The model under review builds one solid part; all positions refer to its coordinate system, in mm. Face numbers are marked on the shaded views. A direction names the side the tool comes from. Give positions to 0.01 mm unless a question says otherwise; leave off trailing zeros. Write each loop counter-clockwise with the first axis right and the second up, starting at its lowest first coordinate (ties: lowest second). Pieces come first, ordered by that corner, then holes. Notation, with made-up numbers: (-26.75, 31.25) - (7.25, 31.25) arc R24 ccw to (7.25, 67.25) - close; hole circle Ø3 at (8, 46.5). An arc over 180 degrees is marked (long way). Write item = value, one per line.
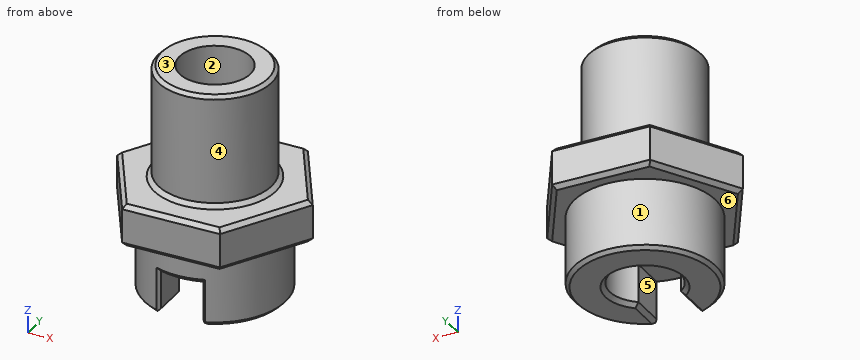
```python
from build123d import *

# Parameters (mm, degrees)
SKETCH1_R           = 4
BOSS_EXTRUDE1_DEPTH = 8
BOSS_EXTRUDE2_DEPTH = 3
SKETCH3_R           = 5
BOSS_EXTRUDE3_DEPTH = 5
SKETCH4_R           = 2.5
CUT_EXTRUDE1_DEPTH  = 19.439088915
CHAMFER1_SIZE       = 0.3
CHAMFER2_SIZE       = 0.3
SKETCH5_W           = 3
SKETCH5_H           = 3
CUT_EXTRUDE2_DEPTH  = 13.165525061
CHAMFER3_SIZE       = 0.3
CHAMFER4_SIZE       = 0.3
CHAMFER5_SIZE       = 0.25


with BuildPart() as part:
    # Sketch1 → Boss-Extrude1 (new body)
    with BuildSketch(Plane.XY):
        Circle(SKETCH1_R)
    extrude(amount=BOSS_EXTRUDE1_DEPTH)

    # Sketch2 → Boss-Extrude2 (add)
    with BuildSketch(Plane(origin=(0, 0, 0), x_dir=(-1, 0, 0), z_dir=(0, 0, -1))):
        Polygon((-3.464101615, 6), (-6.92820323, 0), (-3.464101615, -6), (3.464101615, -6), (6.92820323, 0), (3.464101615, 6), align=None)
    extrude(amount=BOSS_EXTRUDE2_DEPTH)

    # Sketch3 → Boss-Extrude3 (add)
    with BuildSketch(Plane(origin=(0, 0, -3), x_dir=(-1, 0, 0), z_dir=(0, 0, -1))):
        Circle(SKETCH3_R)
    extrude(amount=BOSS_EXTRUDE3_DEPTH)

    # Sketch4 → Cut-Extrude1 (cut, through all)
    with BuildSketch(Plane.XY.offset(8)):
        Circle(SKETCH4_R)
    extrude(amount=-CUT_EXTRUDE1_DEPTH, mode=Mode.SUBTRACT)

    # Chamfer1
    chamfer1_edges = [part.edges().sort_by_distance(p)[0] for p in [
        (-4, 0, 0),
    ]]
    chamfer(chamfer1_edges, length=CHAMFER1_SIZE)

    # Chamfer2
    chamfer2_edges = [part.edges().sort_by_distance(p)[0] for p in [
        (-2.5, 0, -8),
    ]]
    chamfer(chamfer2_edges, length=CHAMFER2_SIZE)

    # Sketch5 → Cut-Extrude2 (cut, through all)
    with BuildSketch(Plane(origin=(0, 0, 0), x_dir=(1, 0, 0), z_dir=(0, 1, 0))):
        with Locations((0, 6.5)):
            Rectangle(SKETCH5_W, SKETCH5_H)
    extrude(amount=-CUT_EXTRUDE2_DEPTH, mode=Mode.SUBTRACT)

    # Chamfer3
    chamfer3_edges = [part.edges().sort_by_distance(p)[0] for p in [
        (-5.196152423, 3, -3),
        (0, 6, 0),
        (5.196152423, 3, 0),
        (5.196152423, -3, 0),
        (0, -6, 0),
        (-5.196152423, -3, 0),
        (-5.196152423, 3, 0),
        (0, 6, -3),
        (5.196152423, 3, -3),
        (5.196152423, -3, -3),
        (0, -6, -3),
        (-5.196152423, -3, -3),
    ]]
    chamfer(chamfer3_edges, length=CHAMFER3_SIZE)

    # Chamfer4
    # the kernel refuses this chamfer: 0.3, 0.239246049 mm, written as the material it takes off along each edge
    with BuildSketch(Plane(origin=(1.5, -1.592813187, -8), x_dir=(0, 0, 1), z_dir=(0, -1, 0))) as chamfer4_piece_1:
        Polygon((CHAMFER4_SIZE, 0), (0, -CHAMFER4_SIZE), (0, 0), align=None)
    extrude(amount=3.948387716, mode=Mode.SUBTRACT)
    with BuildSketch(Plane(origin=(-1.5, -1.592813187, -8), x_dir=(0, 0, 1), z_dir=(0, -1, 0))) as chamfer4_piece_2:
        Polygon((CHAMFER4_SIZE, 0), (0, CHAMFER4_SIZE), (0, 0), align=None)
    extrude(amount=3.948387716, mode=Mode.SUBTRACT)
    with BuildSketch(Plane(origin=(0, 0, -5), x_dir=(-0.44305448610570786, -0.8964946861758898, 0), z_dir=(-0.8964946861758898, 0.44305448610570786, 0))) as chamfer4_piece_3_section:
        Polygon((5, CHAMFER4_SIZE), (5 - CHAMFER4_SIZE, 0), (5, 0), align=None)
    chamfer4_piece_3 = revolve(axis=Axis((0, 0, -5), (0, 0, 1)), revolution_arc=52.597864763, mode=Mode.PRIVATE)
    chamfer4_piece_3 = split(chamfer4_piece_3, bisect_by=Plane(origin=(1.5, 0, -5), z_dir=(-1, 0, 0)), keep=Keep.TOP, mode=Mode.PRIVATE)
    chamfer4_piece_3 = split(chamfer4_piece_3, bisect_by=Plane(origin=(-1.5, 0, -5), z_dir=(1, 0, 0)), keep=Keep.TOP, mode=Mode.PRIVATE)
    add(chamfer4_piece_3, mode=Mode.SUBTRACT)
    with BuildSketch(Plane(origin=(-1.5, -4.769696007, -8.771504896), x_dir=(-0.946580683310887, 0.32246706805919617, 0), z_dir=(0, 0, 1))) as chamfer4_piece_4:
        with BuildLine():
            Line((0.236397724, 0), (CHAMFER4_SIZE * 0.322467068059, -CHAMFER4_SIZE * 0.946580683311))
            Line((CHAMFER4_SIZE * 0.322467068059, -CHAMFER4_SIZE * 0.946580683311), (0, 0))
            ThreePointArc((0, 0), (0.120844642, 0.001396592), (0.236397724, 0))
        make_face()
    extrude(amount=3.771504896, mode=Mode.SUBTRACT)
    with BuildSketch(Plane(origin=(1.5, -4.769696007, -8.771504896), x_dir=(0.9465806833108867, 0.32246706805919695, 0), z_dir=(0, 0, 1))) as chamfer4_piece_5:
        with BuildLine():
            Line((0.236397724, 0), (CHAMFER4_SIZE * 0.322467068059, CHAMFER4_SIZE * 0.946580683311))
            Line((CHAMFER4_SIZE * 0.322467068059, CHAMFER4_SIZE * 0.946580683311), (0, 0))
            ThreePointArc((0, 0), (0.120844642, -0.001396592), (0.236397724, 0))
        make_face()
    extrude(amount=3.771504896, mode=Mode.SUBTRACT)
    with BuildSketch(Plane(origin=(-1.5, -4.769696007, -8.771504896), x_dir=(-0.946580683310887, 0.32246706805919617, 0), z_dir=(0, 0, 1))) as chamfer4_piece_6a_section:
        with BuildLine():
            Line((0.236397724, 0), (CHAMFER4_SIZE * 0.322467068059, -CHAMFER4_SIZE * 0.946580683311))
            Line((CHAMFER4_SIZE * 0.322467068059, -CHAMFER4_SIZE * 0.946580683311), (0, 0))
            ThreePointArc((0, 0), (0.120844642, 0.001396592), (0.236397724, 0))
        make_face()
    chamfer4_piece_6a = extrude(amount=4.543009793, mode=Mode.PRIVATE)
    chamfer4_piece_6a = split(chamfer4_piece_6a, bisect_by=Plane(origin=(-1.5, -4.769696007, -5), z_dir=(0, 0, 1)), keep=Keep.TOP, mode=Mode.PRIVATE)
    with BuildSketch(Plane(origin=(0, 0, -5), x_dir=(-0.44305448610570786, -0.8964946861758898, 0), z_dir=(-0.8964946861758898, 0.44305448610570786, 0))) as chamfer4_piece_6b_section:
        Polygon((5, CHAMFER4_SIZE), (5 - CHAMFER4_SIZE, 0), (5, 0), align=None)
    chamfer4_piece_6b = revolve(axis=Axis((0, 0, -5), (0, 0, 1)), revolution_arc=52.597864763, mode=Mode.PRIVATE)
    chamfer4_piece_6b = split(chamfer4_piece_6b, bisect_by=Plane(origin=(-1.5, 0, -5), z_dir=(-1, 0, 0)), keep=Keep.TOP, mode=Mode.PRIVATE)
    chamfer4_piece_6 = chamfer4_piece_6a & chamfer4_piece_6b
    add(chamfer4_piece_6, mode=Mode.SUBTRACT)
    with BuildSketch(Plane(origin=(0, 0, -5), x_dir=(-0.44305448610570786, -0.8964946861758898, 0), z_dir=(-0.8964946861758898, 0.44305448610570786, 0))) as chamfer4_piece_7a_section:
        Polygon((5, CHAMFER4_SIZE), (5 - CHAMFER4_SIZE, 0), (5, 0), align=None)
    chamfer4_piece_7a = revolve(axis=Axis((0, 0, -5), (0, 0, 1)), revolution_arc=52.597864763, mode=Mode.PRIVATE)
    chamfer4_piece_7a = split(chamfer4_piece_7a, bisect_by=Plane(origin=(1.5, 0, -5), z_dir=(1, 0, 0)), keep=Keep.TOP, mode=Mode.PRIVATE)
    with BuildSketch(Plane(origin=(1.5, -4.769696007, -8.771504896), x_dir=(0.9465806833108867, 0.32246706805919695, 0), z_dir=(0, 0, 1))) as chamfer4_piece_7b_section:
        with BuildLine():
            Line((0.236397724, 0), (CHAMFER4_SIZE * 0.322467068059, CHAMFER4_SIZE * 0.946580683311))
            Line((CHAMFER4_SIZE * 0.322467068059, CHAMFER4_SIZE * 0.946580683311), (0, 0))
            ThreePointArc((0, 0), (0.120844642, -0.001396592), (0.236397724, 0))
        make_face()
    chamfer4_piece_7b = extrude(amount=4.543009793, mode=Mode.PRIVATE)
    chamfer4_piece_7b = split(chamfer4_piece_7b, bisect_by=Plane(origin=(1.5, -4.769696007, -5), z_dir=(0, 0, 1)), keep=Keep.TOP, mode=Mode.PRIVATE)
    chamfer4_piece_7 = chamfer4_piece_7a & chamfer4_piece_7b
    add(chamfer4_piece_7, mode=Mode.SUBTRACT)

    # Chamfer5
    chamfer5_edges = [part.edges().sort_by_distance(p)[0] for p in [
        (2.828427125, 4.123105626, -8),
        (-4, 0, 8),
    ]]
    chamfer(chamfer5_edges, length=CHAMFER5_SIZE)


solid = part.part
```
1. Take a section at C-C on z = -6.25. Give the boundary of the cut face in (x, y).
Findings below:
outline = (-1.72, -4.69) - (-1.5, -4.47) - (-1.5, -2) arc R2.5 cw (long way) to (1.5, -2) - (1.5, -4.47) - (1.72, -4.69) arc R5 ccw (long way) to start
2. Take a section at B-B on z = -1.25. Give the boundary of the cut face in (x, y), and give its area (3 significant figures).
Findings below:
outline = (-6.93, 0) - (-3.46, -6) - (3.46, -6) - (6.93, 0) - (3.46, 6) - (-3.46, 6) - close; hole circle Ø5 at (0, 0)
area = 105 mm²
3. Insertion check: P1, Ø6, axis at x = 1.5, z = 2.5, coming from the -Y side; P2, Ø2, axis at y = -3.5, z = -6, coming from the +X side; P3, Ø2.5, axis at y = -4, z = -6, coming from the -X side; P4, Ø0.8, axis at x = -0.5, y = -4, coming from the -Z side. Each pin has a flat end and moves straight along its axis. Give the tip position at first contact, or say it passes through.
Findings below:
P1 = -6
P2 = 4.33
P3 = -4.18
P4 = -5
4. Take a section at A-A on x = 0. Give the boundary of the cut face in (y, z).
Findings below:
outline = (-6, -2.7) - (-5.7, -3) - (-5, -3) - (-5, -4.7) - (-4.7, -5) - (-2.5, -5) - (-2.5, 8) - (-3.75, 8) - (-4, 7.75) - (-4, 0.3) - (-4.3, 0) - (-5.7, 0) - (-6, -0.3) - close; (2.5, -7.7) - (2.8, -8) - (4.75, -8) - (5, -7.75) - (5, -3) - (5.7, -3) - (6, -2.7) - (6, -0.3) - (5.7, 0) - (4.3, 0) - (4, 0.3) - (4, 7.75) - (3.75, 8) - (2.5, 8) - close
5. Take a section at D-D on x = -6. Give the boundary of the cut face in (y, z), and give its area (3 significant figures).
Findings below:
outline = (-1.61, -2.7) - (-1.01, -3) - (1.01, -3) - (1.61, -2.7) - (1.61, -0.3) - (1.01, 0) - (-1.01, 0) - (-1.61, -0.3) - close
area = 9.29 mm²
6. For line 1 (Y direction, x = 0, z = -3.5); line 2 (Y direction, x = 0, z = 4.25); line 3 (X direction, y = 2, z = 3), list the stretches that pass through material, from the lowest coordinate up. Write a range as from..to.
Findings below:
line_1 = -5..-2.5, 2.5..5
line_2 = -4..-2.5, 2.5..4
line_3 = -3.46..-1.5, 1.5..3.46
7. Draft analysis for pull direction Y (two halves, no side actions). For the marked faces 1, 2 and 3, state which applies: +Y half, -Y half, draft (parallel to the pull), parting line (faces both ways), or undercut.
Findings below:
face_1 = parting line
face_2 = undercut
face_3 = draft
8. Machinability: for the marked faces 4, 5 and 6, which of the approach directions +Z, -Z, +X, -X, +Y, -Y give a long, thin tool a straight path to every point of the face, cutting with its end or side? Answer none if there is none.
Findings below:
face_4 = +Z
face_5 = -Z, -Y
face_6 = -Z
